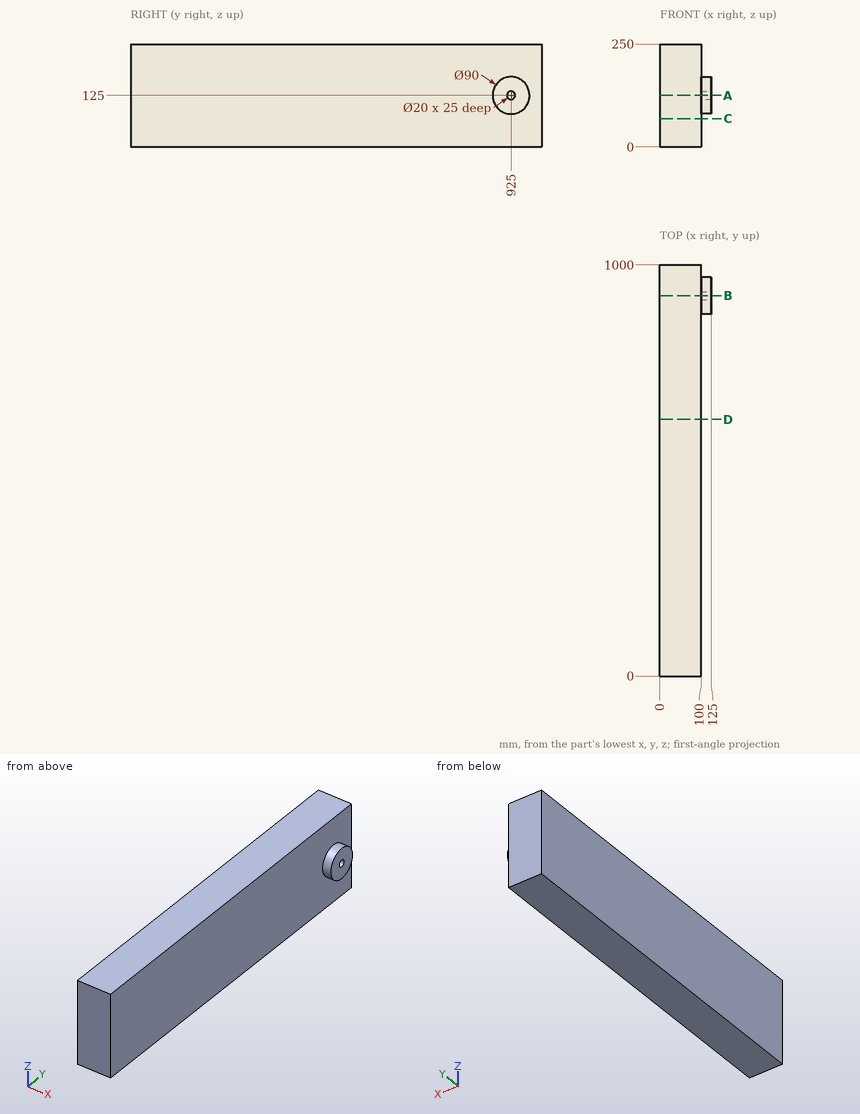
Input: dimensioned drawing with shaded views. Units: mm. Origin: part minimum x, y, z. Give positions to 0.01 mm unless a question says otherwise; leave off trailing zeros. Write each loop counter-clockwise with the first axis right and the second up, starting at its lowest first coordinate (ties: lowest second). Pieces come first, ordered by that corner, then holes.
1. Section query D-D (y = 624). Return the cut outline in (x, z), then the cut area to 3 significant figures.
2. Material intervals for line 1 along Y through (x, z) = (120, 125); line 2 along Z through (x, y) = (117, 925); line 3 along X through (y, z) = (238, 28), sorted ascending.
3. Section query C-C (z = 68.5). Return the cut outline in (x, y).
4. First-contact query: pin 1 (5 mm diameter, centred on y = 691, z = 143.5, fed in from +X); pin 2 (8 mm diameter, centred on y = 242, z = 222.5, fed in from -X). Flat tips, straight axial feed; report the tip coordinate or a pass-through.
5. Section query B-B (y = 925). Return the cut outline in (x, z).
6. Section query A-A (z = 125). Return the cut outline in (x, y), then the cut area to 3 significant figures.
Output values:
1. outline: (0, 0) - (100, 0) - (100, 250) - (0, 250) - close
1. area: 25,000 mm2
2. line 1: y = 880 to 915, 935 to 970
2. line 2: z = 80 to 115, 135 to 170
2. line 3: x = 0 to 100
3. outline: (0, 0) - (100, 0) - (100, 1000) - (0, 1000) - close
4. pin 1: stops at x = 100
4. pin 2: stops at x = 0
5. outline: (0, 0) - (100, 0) - (100, 80) - (125, 80) - (125, 115) - (100, 115) - (100, 135) - (125, 135) - (125, 170) - (100, 170) - (100, 250) - (0, 250) - close
6. outline: (0, 0) - (100, 0) - (100, 880) - (125, 880) - (125, 915) - (100, 915) - (100, 935) - (125, 935) - (125, 970) - (100, 970) - (100, 1000) - (0, 1000) - close
6. area: 102,000 mm2
